Source: three-view drawing plus pictorial views. Frame: mm from the lowest corner of the part. Give positions to 0.01 mm unless a question says otherwise; leave off trailing zeros. Loops run counter-clockwise (first coordinate to the right, second up) from the corner with the lowest first, then second, coordinate; pieces in that order, holes last.
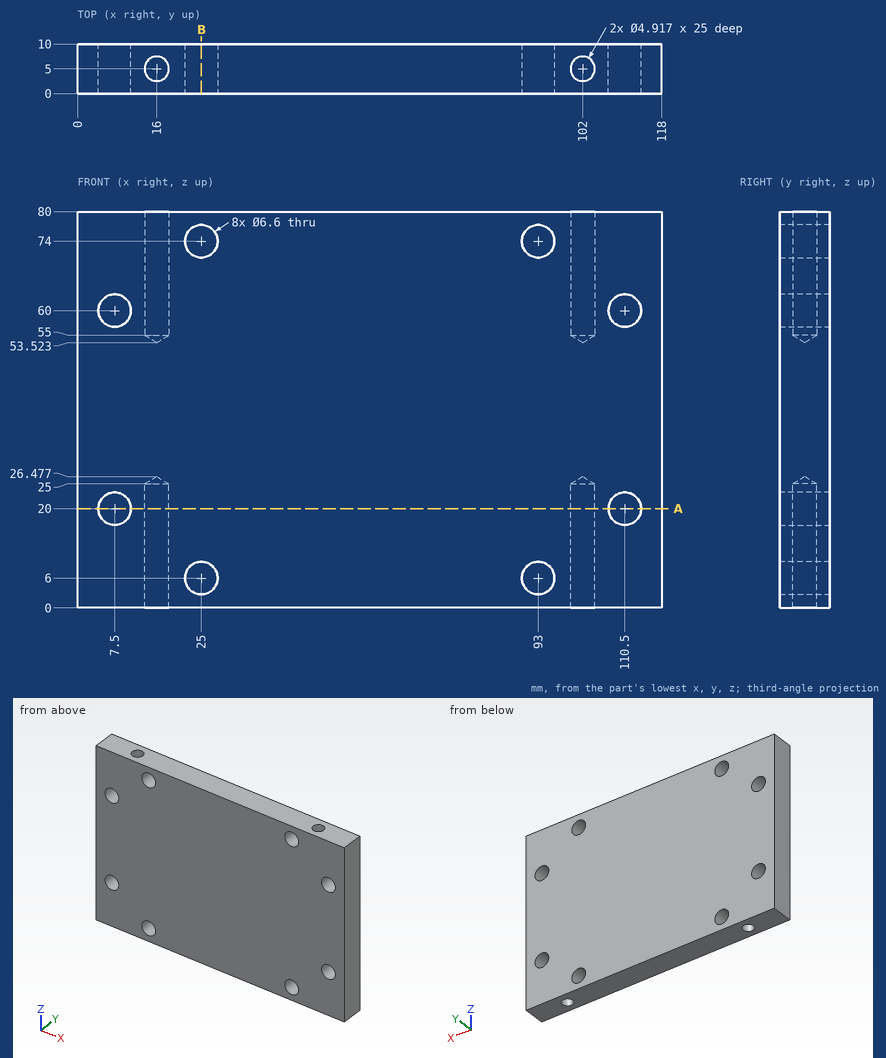
1) Cut plane A-A (z = 20). Return loops of the section in (x, y), and give its area (3 significant figures).
Checks:
outline: (0, 0) - (4.2, 0) - (4.2, 10) - (0, 10) - close; (10.8, 0) - (107.2, 0) - (107.2, 10) - (10.8, 10) - close; (113.8, 0) - (118, 0) - (118, 10) - (113.8, 10) - close; hole circle Ø4.92 at (16, 5); hole circle Ø4.92 at (102, 5)
area: 1,010 mm2
2) Cut plane B-B (x = 25). Return loops of the section in (y, z), and give its area (3 significant figures).
Checks:
outline: (0, 0) - (10, 0) - (10, 2.7) - (0, 2.7) - close; (0, 9.3) - (10, 9.3) - (10, 70.7) - (0, 70.7) - close; (0, 77.3) - (10, 77.3) - (10, 80) - (0, 80) - close
area: 668 mm2
3) Ray query, probe 1 along X at (y, z) = (5, 20); probe 2 along Z at (x, y) = (7.5, 7.25); probe 3 along X at (y, z) = (7.5, 6). Return the intervals inside material, ascending.
Checks:
probe 1: x = 0 to 4.2, 10.8 to 13.54, 18.46 to 99.54, 104.46 to 107.2, 113.8 to 118
probe 2: z = 0 to 16.7, 23.3 to 56.7, 63.3 to 80
probe 3: x = 0 to 21.7, 28.3 to 89.7, 96.3 to 118
4) Contact query for flat-ended pins moving along their axis: P1, Ø4, axis at x = 102, y = 5, coming from the -Z side (1 decimal); P2, Ø4, axis at x = 93, z = 74, coming from the +Y side. Output: stop coordinate, or through.
Checks:
P1: stops at z = 25.3
P2: passes through
